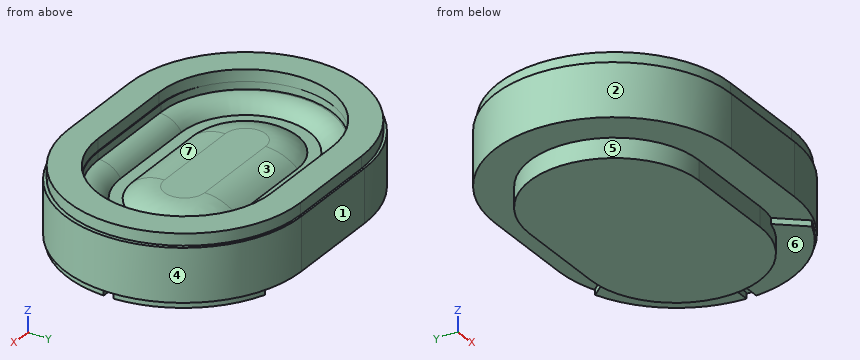
from build123d import *

# Parameters (mm, degrees)
EXTRUDE_1_DEPTH     = 1
EXTRUDE_2_DEPTH     = 2.7
EXTRUDE_1_2_DEPTH   = 0.6
CUT_EXTRUDE_1_DEPTH = 1
CUT_EXTRUDE_2_DEPTH = 0.4
FILLET_1_R          = 1.3
FILLET_2_R          = 2.5
EXTRUDE_START       = -0.3
EXTRUDE_3_DEPTH     = 0.3


with BuildPart() as part:
    # Эскиз1 → Extrude 1 (new body)
    with BuildSketch(Plane.XY):
        with BuildLine():
            Line((-2.4, 4.3), (2.4, 4.3))
            ThreePointArc((2.4, 4.3), (6.7, 0), (2.4, -4.3))
            Line((2.4, -4.3), (-2.4, -4.3))
            ThreePointArc((-2.4, -4.3), (-6.7, 0), (-2.4, 4.3))
        make_face()
    extrude(amount=EXTRUDE_1_DEPTH)

    # Эскиз2 → Бобышка-Вытянуть2 (add)
    with BuildSketch(Plane.XY.offset(1)):
        with BuildLine():
            Line((-2.5, 6), (2.5, 6))
            ThreePointArc((2.5, 6), (8.5, 0), (2.5, -6))
            Line((2.5, -6), (-2.5, -6))
            ThreePointArc((-2.5, -6), (-8.5, 0), (-2.5, 6))
        make_face()
    extrude(amount=EXTRUDE_2_DEPTH)

    # Эскиз3 → Extrude 1 2 (add)
    with BuildSketch(Plane.XY.offset(3.7)):
        with BuildLine():
            Line((2.4, -5.9), (-2.4, -5.9))
            ThreePointArc((-2.4, -5.9), (-8.3, 0), (-2.4, 5.9))
            Line((-2.4, 5.9), (2.4, 5.9))
            ThreePointArc((2.4, 5.9), (8.3, 0), (2.4, -5.9))
        make_face()
        with BuildLine():
            Line((2.4, -4.4), (-2.4, -4.4))
            ThreePointArc((-2.4, -4.4), (-6.8, 0), (-2.4, 4.4))
            Line((-2.4, 4.4), (2.4, 4.4))
            ThreePointArc((2.4, 4.4), (6.8, 0), (2.4, -4.4))
        make_face(mode=Mode.SUBTRACT)
    extrude(amount=EXTRUDE_1_2_DEPTH)

    # Эскиз4 → Вырез-Вытянуть1 (cut)
    with BuildSketch(Plane.XY.offset(3.7)):
        with BuildLine():
            Line((-2.4, 3.25), (2.4, 3.25))
            ThreePointArc((2.4, 3.25), (5.65, 0), (2.4, -3.25))
            Line((2.4, -3.25), (-2.4, -3.25))
            ThreePointArc((-2.4, -3.25), (-5.65, 0), (-2.4, 3.25))
        make_face()
        with BuildLine():
            Line((2.4, -2.65), (-2.4, -2.65))
            ThreePointArc((-2.4, -2.65), (-5.05, 0), (-2.4, 2.65))
            Line((-2.4, 2.65), (2.4, 2.65))
            ThreePointArc((2.4, 2.65), (5.05, 0), (2.4, -2.65))
        make_face(mode=Mode.SUBTRACT)
    extrude(amount=-CUT_EXTRUDE_1_DEPTH, mode=Mode.SUBTRACT)

    # Эскиз5 → Вырез-Вытянуть2 (cut)
    with BuildSketch(Plane.XY.offset(3.7)):
        with BuildLine():
            Line((2.5, -4.35), (-2.5, -4.35))
            ThreePointArc((-2.5, -4.35), (-6.85, 0), (-2.5, 4.35))
            Line((-2.5, 4.35), (2.5, 4.35))
            ThreePointArc((2.5, 4.35), (6.85, 0), (2.5, -4.35))
        make_face()
    extrude(amount=-CUT_EXTRUDE_2_DEPTH, mode=Mode.SUBTRACT)

    # Скругление1
    # the kernel refuses this fillet: 1.3 mm, written as the material it takes off along each edge
    with BuildSketch(Plane(origin=(2.4, 0, 3.3), x_dir=(0, -1, 0), z_dir=(-1, 0, 0))) as fillet_1_piece_1:
        with BuildLine():
            CenterArc((4.345445115, -1.3), FILLET_1_R, 90, 57.421029607)
            Line((3.25, -0.6), (3.25, 0))
            Line((3.25, 0), (4.345445115, 0))
        make_face()
    revolve(axis=Axis((2.4, 0, 3.3), (0, 0, 1)), revolution_arc=180, mode=Mode.SUBTRACT)
    with BuildSketch(Plane(origin=(-2.4, 3.25, 3.3), x_dir=(0, 1, 0), z_dir=(1, 0, 0)), Plane(origin=(2.4, -3.25, 3.3), x_dir=(0, -1, 0), z_dir=(-1, 0, 0))) as fillet_1_piece_2:
        with BuildLine():
            CenterArc((1.095445115, -1.3), FILLET_1_R, 90, 57.421029607)
            Line((0, -0.6), (0, 0))
            Line((0, 0), (1.095445115, 0))
        make_face()
    extrude(amount=4.8, mode=Mode.SUBTRACT)
    with BuildSketch(Plane(origin=(-2.4, 0, 3.3), x_dir=(0, 1, 0), z_dir=(1, 0, 0))) as fillet_1_piece_3:
        with BuildLine():
            CenterArc((4.345445115, -1.3), FILLET_1_R, 90, 57.421029607)
            Line((3.25, -0.6), (3.25, 0))
            Line((3.25, 0), (4.345445115, 0))
        make_face()
    revolve(axis=Axis((-2.4, 0, 3.3), (0, 0, 1)), revolution_arc=180, mode=Mode.SUBTRACT)

    # Скругление2
    # the kernel refuses this fillet: 2.5 mm, written as the material it takes off along each edge
    with BuildSketch(Plane(origin=(2.4, 0, 3.3), x_dir=(0, -1, 0), z_dir=(-1, 0, 0))) as fillet_2_piece_1:
        with BuildLine():
            CenterArc((1.025192319, -2.5), FILLET_2_R, 49.464197889, 40.535802111)
            Line((1.025192319, 0), (1.025192319, 0.05))
            Line((1.025192319, 0.05), (2.65, 0.05))
            Line((2.65, 0.05), (2.7, 0))
            ThreePointArc((2.7, 0), (2.7, -0.3), (2.682496154, -0.562))
            Line((2.682496154, -0.562), (2.65, -0.6))
        make_face()
    revolve(axis=Axis((2.4, 0, 3.3), (0, 0, 1)), revolution_arc=180, mode=Mode.SUBTRACT)
    with BuildSketch(Plane(origin=(-2.4, 2.65, 3.3), x_dir=(0, 0, -1), z_dir=(1, 0, 0)), Plane(origin=(2.4, -2.65, 3.3), x_dir=(0, 0, -1), z_dir=(-1, 0, 0))) as fillet_2_piece_2:
        with BuildLine():
            CenterArc((2.5, -1.624807681), FILLET_2_R, 139.464197889, 40.535802111)
            Line((0, -1.624807681), (-0.05, -1.624807681))
            Line((-0.05, -1.624807681), (-0.05, 0))
            Line((-0.05, 0), (0, 0.05))
            ThreePointArc((0, 0.05), (0.3, 0.05), (0.562, 0.032496154))
            Line((0.562, 0.032496154), (0.6, 0))
        make_face()
    extrude(amount=4.8, mode=Mode.SUBTRACT)
    with BuildSketch(Plane(origin=(-2.4, 0, 3.3), x_dir=(0, 1, 0), z_dir=(1, 0, 0))) as fillet_2_piece_3:
        with BuildLine():
            CenterArc((1.025192319, -2.5), FILLET_2_R, 49.464197889, 40.535802111)
            Line((1.025192319, 0), (1.025192319, 0.05))
            Line((1.025192319, 0.05), (2.65, 0.05))
            Line((2.65, 0.05), (2.7, 0))
            ThreePointArc((2.7, 0), (2.7, -0.3), (2.682496154, -0.562))
            Line((2.682496154, -0.562), (2.65, -0.6))
        make_face()
    revolve(axis=Axis((-2.4, 0, 3.3), (0, 0, 1)), revolution_arc=180, mode=Mode.SUBTRACT)

    # Эскиз6 → Бобышка-Вытянуть3 (add)
    with BuildSketch(Plane.XY.offset(1).offset(EXTRUDE_START)):
        with BuildLine():
            Line((6.692726406, 0.25), (8.40002281, 0.25))
            ThreePointArc((8.40002281, 0.25), (7.297123742, 3.443889221), (4.623650475, 5.510252065))
            Line((4.623650475, 5.510252065), (3.490230582, 4.159494835))
            ThreePointArc((3.490230582, 4.159494835), (5.726423597, 2.72486808), (6.692726406, 0.25))
        make_face()
        with BuildLine():
            Line((6.692726406, -0.25), (8.40002281, -0.25))
            ThreePointArc((8.40002281, -0.25), (7.297123742, -3.443889221), (4.623650475, -5.510252065))
            Line((4.623650475, -5.510252065), (3.490230582, -4.159494835))
            ThreePointArc((3.490230582, -4.159494835), (5.726423597, -2.72486808), (6.692726406, -0.25))
        make_face()
    extrude(amount=EXTRUDE_3_DEPTH)


solid = part.part
Check sheet for the modelled part. Datum: model origin and axes. Units: mm. Face numbers are marked on the shaded views. A direction names the side the tool comes from. Coordinates: 2 decimals unless noted, no trailing zeros. Loops run counter-clockwise (first coordinate to the right, second up) from the corner with the lowest first, then second, coordinate; pieces in that order, holes last. Notation, with made-up numbers: (6, 15) -> (37, 15) arc R29 ccw to (37, 36) -> close; hole circle Ø1 at (-16, 29). An arc over 180 degrees is marked (long way). Answer in a Markdown table with one row per item.
1. Sectioned sample at C-C, the plane y = -4.75. Record the boundary of the cut face in (x, z).
Check values:
| item | result |
|---|---|
| outline | (-6.17, 1) -> (3.99, 1) -> (3.99, 0.7) -> (6.01, 0.7) -> (6.01, 1) -> (6.17, 1) -> (6.17, 3.7) -> (5.9, 3.7) -> (5.9, 4.3) -> (-5.9, 4.3) -> (-5.9, 3.7) -> (-6.17, 3.7) -> close |
2. Release check for a two-part mould opening along X. For the marked faces 1, 2, 3 and 4 record: released by +X, released by -X, zero draft, split by the parting line, or undercut.
Check values:
| item | result |
|---|---|
| face 1 | zero draft |
| face 2 | released by -X |
| face 3 | undercut |
| face 4 | released by +X |
3. Go/stop test with flat-tipped pins: pin 1 (0.5 mm diameter, centred on x = -1, z = 4, fed in from -Y); pin 2 (0.5 mm diameter, centred on x = -1, z = 4, fed in from +Y); pin 3 (1.5 mm diameter, centred on y = 1.5, z = 2.5, fed in from -X). Record where each tip stops, or that it passes through.
Check values:
| item | result |
|---|---|
| pin 1 | stops at y = -5.9 |
| pin 2 | stops at y = 5.9 |
| pin 3 | stops at x = -8.45 |
4. Sectioned sample at A-A, the plane y = 5. Record the boundary of the cut face in (x, z).
Check values:
| item | result |
|---|---|
| outline | (-5.82, 1) -> (4.2, 1) -> (4.2, 0.7) -> (5.64, 0.7) -> (5.64, 1) -> (5.82, 1) -> (5.82, 3.7) -> (5.53, 3.7) -> (5.53, 4.3) -> (-5.53, 4.3) -> (-5.53, 3.7) -> (-5.82, 3.7) -> close |
5. Access from +Z, -Z, +X, -X, +Y, -Y to the whole of each face (thin tool, end or side, straight path). Record for the marked faces 5, 6 and 7.
Check values:
| item | result |
|---|---|
| face 5 | -Z, -X |
| face 6 | -Z, +X, -Y |
| face 7 | +Z |
6. Material ranges on line 1 along Y through (x, z) = (-1.5, 4.05); line 2 along Y through (x, z) = (-0.5, 3); line 3 along X through (y, z) = (1.5, 2.85), recorded low to high. Write a range as [from, to].
Check values:
| item | result |
|---|---|
| line 1 | y = [-5.9, -4.4], [4.4, 5.9] |
| line 2 | y = [-6, -3.51], [-2.21, 2.21], [3.51, 6] |
| line 3 | x = [-8.31, -5.41], [-4.34, 4.34], [5.41, 8.31] |
7. Sectioned sample at B-B, the plane z = 1.9. Record the boundary of the cut face in (x, y), then the cut area to 3 significant figures.
Check values:
| item | result |
|---|---|
| outline | (-2.5, -6) -> (2.5, -6) arc R6 ccw to (2.5, 6) -> (-2.5, 6) arc R6 ccw to start |
| area | 173 mm2 |
